```python
from build123d import *

# Parameters (mm, degrees)
SKETCH_W        = 100
SKETCH_H        = 42
PAD_DEPTH       = 12
POCKET_DEPTH    = 3
POCKET001_DEPTH = 7.5
SKETCH002_W     = 14
SKETCH002_H     = 7
POCKET002_DEPTH = 5
SKETCH004_W     = 7
SKETCH004_H     = 6
POCKET003_DEPTH = 5
SKETCH005_W     = 10
SKETCH005_H     = 4
POCKET004_DEPTH = 5
FILLET_R        = 4
FILLET001_R     = 4
FILLET002_R     = 1
FILLET003_R     = 1
FILLET004_R     = 4
FILLET005_R     = 1
FILLET006_R     = 1


with BuildPart() as part:
    # Sketch → Pad (new body)
    with BuildSketch(Plane.XY):
        Rectangle(SKETCH_W, SKETCH_H)
        Polygon((-44.412287, 14.25), (-42.824574, 17), (-44.412287, 19.75), (-47.587713, 19.75), (-49.175426, 17), (-47.587713, 14.25), align=None, mode=Mode.SUBTRACT)
        Polygon((-44.412287, -19.75), (-42.824574, -17), (-44.412287, -14.25), (-47.587713, -14.25), (-49.175426, -17), (-47.587713, -19.75), align=None, mode=Mode.SUBTRACT)
        Polygon((49.175426, 17), (47.587713, 19.75), (44.412287, 19.75), (42.824574, 17), (44.412287, 14.25), (47.587713, 14.25), align=None, mode=Mode.SUBTRACT)
        Polygon((47.587713, -19.75), (49.175426, -17), (47.587713, -14.25), (44.412287, -14.25), (42.824574, -17), (44.412287, -19.75), align=None, mode=Mode.SUBTRACT)
    extrude(amount=PAD_DEPTH)

    # Sketch001 → Pocket (cut)
    with BuildSketch(Plane.XY.offset(12)):
        Polygon((-48, 13), (-48, -13), (-42, -13), (-42, -19), (42, -19), (42, -13), (48, -13), (48, 13), (42, 13), (42, 19), (-42, 19), (-42, 13), align=None)
    extrude(amount=-POCKET_DEPTH, mode=Mode.SUBTRACT)

    # Sketch003 → Pocket001 (cut)
    with BuildSketch(Plane(origin=(0, 0, 0), x_dir=(1, 0, 0), z_dir=(0, 0, -1))):
        Polygon((-48, 13), (-48, -13), (-42, -13), (-42, -19), (42, -19), (42, -13), (48, -13), (48, 13), (42, 13), (42, 19), (-42, 19), (-42, 13), align=None)
    extrude(amount=-POCKET001_DEPTH, mode=Mode.SUBTRACT)

    # Sketch002 → Pocket002 (cut)
    with BuildSketch(Plane.XY.offset(9)):
        with Locations((0, -12.5)):
            Rectangle(SKETCH002_W, SKETCH002_H)
    extrude(amount=-POCKET002_DEPTH, mode=Mode.SUBTRACT)

    # Sketch004 → Pocket003 (cut)
    with BuildSketch(Plane.XZ.offset(21)):
        with Locations((21, 3)):
            Rectangle(SKETCH004_W, SKETCH004_H)
    extrude(amount=-POCKET003_DEPTH, mode=Mode.SUBTRACT)

    # Sketch005 → Pocket004 (cut)
    with BuildSketch(Plane.XZ.offset(21)):
        with Locations((32, 2)):
            Rectangle(SKETCH005_W, SKETCH005_H)
    extrude(amount=-POCKET004_DEPTH, mode=Mode.SUBTRACT)

    # Fillet
    fillet_edges = [part.edges().sort_by_distance(p)[0] for p in [
        (50, -21, 6),
        (50, 21, 6),
        (-50, -21, 6),
        (-50, 21, 6),
    ]]
    fillet(fillet_edges, radius=FILLET_R)

    # Fillet001
    fillet001_edges = [part.edges().sort_by_distance(p)[0] for p in [
        (-42, 19, 10.5),
        (48, 13, 10.5),
        (42, -19, 10.5),
        (-48, -13, 10.5),
    ]]
    fillet(fillet001_edges, radius=FILLET001_R)

    # Fillet002
    fillet002_edges = [part.edges().sort_by_distance(p)[0] for p in [
        (42, 19, 10.5),
        (-42, 13, 10.5),
        (42, 13, 10.5),
        (48, -13, 10.5),
        (42, -13, 10.5),
        (-42, -19, 10.5),
        (-42, -13, 10.5),
        (-48, 13, 10.5),
    ]]
    fillet(fillet002_edges, radius=FILLET002_R)

    # Fillet003
    fillet003_edges = [part.edges().sort_by_distance(p)[0] for p in [
        (42, 16, 9),
        (41.707107, 18.707107, 9),
        (1.5, 19, 9),
        (-40.828427, 17.828427, 9),
        (-42, 14.5, 9),
        (-42.292893, 13.292893, 9),
        (-45, 13, 9),
        (-47.707107, 12.707107, 9),
        (-48, 1.5, 9),
        (-46.828427, -11.828427, 9),
        (-43.5, -13, 9),
        (-42.292893, -13.292893, 9),
        (-42, -16, 9),
        (-41.707107, -18.707107, 9),
        (-1.5, -19, 9),
        (40.828427, -17.828427, 9),
        (42.292893, -13.292893, 9),
        (45, -13, 9),
        (42, -14.5, 9),
        (47.707107, -12.707107, 9),
        (48, -1.5, 9),
        (46.828427, 11.828427, 9),
        (43.5, 13, 9),
        (42.292893, 13.292893, 9),
    ]]
    fillet(fillet003_edges, radius=FILLET003_R)

    # Fillet004
    fillet004_edges = [part.edges().sort_by_distance(p)[0] for p in [
        (-42, 13, 3.75),
        (-42, -13, 3.75),
        (42, 13, 3.75),
        (42, -13, 3.75),
    ]]
    fillet(fillet004_edges, radius=FILLET004_R)

    # Fillet005
    fillet005_edges = [part.edges().sort_by_distance(p)[0] for p in [
        (42, -19, 3.75),
        (48, -13, 3.75),
        (48, 13, 3.75),
        (42, 19, 3.75),
        (-42, 19, 3.75),
        (-48, 13, 3.75),
        (-42, -19, 3.75),
        (-48, -13, 3.75),
    ]]
    fillet(fillet005_edges, radius=FILLET005_R)

    # Fillet006
    fillet006_edges = [part.edges().sort_by_distance(p)[0] for p in [
        (0, -19, 7.5),
        (-41.707107, -18.707107, 7.5),
        (-42, -17.5, 7.5),
        (-43.171573, -14.171573, 7.5),
        (-46.5, -13, 7.5),
        (-47.707107, -12.707107, 7.5),
        (-48, 0, 7.5),
        (41.707107, -18.707107, 7.5),
        (42, -17.5, 7.5),
        (43.171573, -14.171573, 7.5),
        (46.5, -13, 7.5),
        (47.707107, -12.707107, 7.5),
        (48, 0, 7.5),
        (47.707107, 12.707107, 7.5),
        (46.5, 13, 7.5),
        (43.171573, 14.171573, 7.5),
        (42, 17.5, 7.5),
        (41.707107, 18.707107, 7.5),
        (0, 19, 7.5),
        (-47.707107, 12.707107, 7.5),
        (-46.5, 13, 7.5),
        (-43.171573, 14.171573, 7.5),
        (-42, 17.5, 7.5),
        (-41.707107, 18.707107, 7.5),
    ]]
    fillet(fillet006_edges, radius=FILLET006_R)


solid = part.part
```
Read the model definition and answer for the solid it produces. Units are mm, in the model's axes. A direction names the side the tool comes from. Give positions to 0.01 mm unless a question says otherwise; leave off trailing zeros. Write each loop counter-clockwise with the first axis right and the second up, starting at its lowest first coordinate (ties: lowest second). Pieces come first, ordered by that corner, then holes. Notation, with made-up numbers: M 8,27.5 L 59,27.5 A12 ccw 59,50.5 Z; hole C 7,58.5 d6. An arc over 180 degrees is marked long. Put each result on its own line as item: value. Start each with the question number.
1. The part is cut by section C-C, the plane y = -5.5. Give the vertices of the cut face in (x, z).
2. The part is cut by section B-B, the plane z = 1.5. Give the number of separate pieces and of enclosed holes in the cut face, and give its area (3 significant figures).
3. The part is cut by section D-D, the plane x = -20.5. Give the vertices of the cut face in (y, z), and give its area (3 significant figures).
4. Which of the six approach directions +Z, -Z, +X, -X, +Y, -Y give full straight-line access (tool end or side, diameter ignored) to faces 1 (the flat face through (43.61, 15.64, 5.92)), 2 (the flat face through (24.5, -20, 3)), 3 (the cylindrical face through (46.859, 11.797, 10.986))?
5. For a pull along Y with two mould halves and no side action, classify faces 4 (the flat face through (-46, 14.25, 6)), 5 (the flat face through (37, -20, 2)), 6 (the flat face through (46, -14.25, 6)) as released by +Y, released by -Y, zero draft, split by the parting line, or undercut.
6. The part is cut by section A-A, the plane x = -4.5. Give the vertices of the cut face in (y, z), and give its area (3 significant figures).
7. Each of these flat-tipped pins is pushed along its axis until it touches: pin 1 Ø1 at (x, z) = (-46.5, 6.5) entering from +Y; pin 2 Ø2 at (y, z) = (-19.5, 4) entering from +X; pin 3 Ø6 at (x, y) = (-37, -11) entering from +Z; pin 4 Ø6 at (x, y) = (-14, -2) entering from -Z. Where does it stop, or does it pass through?
8. Consider line 1 along Y through (x, z) = (-7, 10.75); line 2 along X through (y, z) = (9.5, 2); line 3 along X through (y, z) = (-15, 10.75). Determine where each line is inside the solid, lowest interval first.
Final values:
1. outline: M -50,0 L -48,0 L -48,6.5 A1 cw -47,7.5 L 47,7.5 A1 cw 48,6.5 L 48,0 L 50,0 L 50,12 L 48,12 L 48,10 A1 cw 47,9 L -47,9 A1 cw -48,10 L -48,12 L -50,12 Z
2. separate pieces: 2
2. enclosed holes: 4
2. area: 531 mm²
3. outline: M -21,0 L -19,0 L -19,6.5 A1 cw -18,7.5 L 18,7.5 A1 cw 19,6.5 L 19,0 L 21,0 L 21,12 L 19,12 L 19,10 A1 cw 18,9 L -18,9 A1 cw -19,10 L -19,12 L -21,12 Z
3. area: 106 mm²
4. face 1: +Z, -Z
4. face 2: -Z, -Y
4. face 3: +Z
5. face 4: undercut
5. face 5: zero draft
5. face 6: undercut
6. outline: M -21,0 L -19,0 L -19,6.5 A1 cw -18,7.5 L -16,7.5 L -16,9 L -18,9 A1 cw -19,10 L -19,12 L -21,12 Z; M -9,7.5 L 18,7.5 A1 cw 19,6.5 L 19,0 L 21,0 L 21,12 L 19,12 L 19,10 A1 cw 18,9 L -9,9 Z
6. area: 95.4 mm²
7. pin 1: stops at y = 21
7. pin 2: stops at x = 49.71
7. pin 3: stops at z = 9
7. pin 4: stops at z = 7.5
8. line 1: y = -21 to -19, 19 to 21
8. line 2: x = -50 to -48, 48 to 50
8. line 3: x = -50 to -48.02, -43.98 to -42, 42 to 43.98, 48.02 to 50
